Check sheet for the modelled part. Datum: model origin and axes. Units: mm. Face numbers are marked on the shaded views. A direction names the side the tool comes from. Coordinates: 2 decimals unless noted, no trailing zeros. Write each loop counter-clockwise with the first axis right and the second up, starting at its lowest first coordinate (ties: lowest second). Pieces come first, ordered by that corner, then holes. Notation, with made-up numbers: M 15.5,50.25 L 37.5,50.25 A25 ccw 37.5,88.25 Z; hole C 66,49 d4. An arc over 180 degrees is marked long. Answer as CSV lines item,"result". Start each with the question number.
1) Section check C-C (z = 3). Record the cut outline in (x, y), and give its area (3 significant figures).
2) Access from +Z, -Z, +X, -X, +Y, -Y to the whole of each face (thin tool, end or side, straight path). Record for the marked faces 1, 2 and 3.
3) Draft check along X on the marked faces 4, 5 and 6. Enter one of: +X half, -X half, draft (parallel to the pull), parting line (faces both ways), or undercut.
4) Go/stop test with flat-tipped pins: pin 1 Ø1 at (x, z) = (0.5, 3) entering from +Y; pin 2 Ø2 at (x, y) = (-2.5, 3) entering from +Z; pin 3 Ø1.2 at (x, y) = (0, 0) entering from +Z. Record where each tip stops, or that it passes through.
5) Section check A-A (y = 0). Record the cut outline in (x, z).
6) Material ranges on L1, parallel to Y at x = 0, z = 1.75; L2, parallel to Y at x = 0, z = 0.5, recorded low to high. Write a range as [from, to].
7) Section check D-D (y = -1.25). Record the cut outline in (x, z), and give its area (3 significant figures).
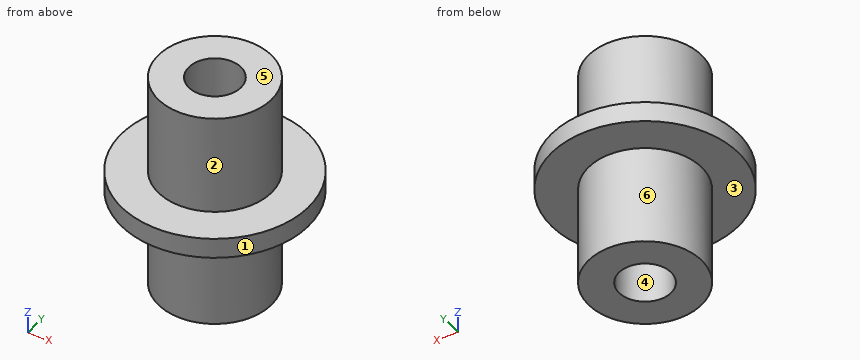
from build123d import *

# Parameters (mm, degrees)
F0_R     = 3.7338
F1_DEPTH = 0.8128
F2_R     = 2.2606
F3_DEPTH = 3.9878
F4_R     = 2.2606
F5_DEPTH = 3.9878
F6_R     = 1.0414
F7_DEPTH = 25.4


with BuildPart() as f1:
    # F0 (on Top) → F1 (new body)
    with BuildSketch(Plane.XY):
        Circle(F0_R)
    extrude(amount=F1_DEPTH)

    # F2 (on face) → F3 (join)
    with BuildSketch(Plane.XY.offset(0.8128)):
        Circle(F2_R)
    extrude(amount=F3_DEPTH)

    # F4 (on face) → F5 (join)
    with BuildSketch(Plane(origin=(0, 0, 0), x_dir=(1, 0, 0), z_dir=(0, 0, -1))):
        Circle(F4_R)
    extrude(amount=F5_DEPTH)

    # F6 (on face) → F7 (cut)
    with BuildSketch(Plane(origin=(0, 0, -3.9878), x_dir=(1, 0, 0), z_dir=(0, 0, -1))):
        Circle(F6_R)
    extrude(amount=-F7_DEPTH, mode=Mode.SUBTRACT)


solid = f1.part
Results found:
1,outline,"C 0,0 d4.52; hole C 0,0 d2.08"
1,area,"12.6 mm2"
2,face 1,"+Z, -Z"
2,face 2,"+Z"
2,face 3,"-Z"
3,face 4,"undercut"
3,face 5,"draft"
3,face 6,"parting line"
4,pin 1,"stops at y = 2.26"
4,pin 2,"stops at z = 0.81"
4,pin 3,"passes through"
5,outline,"M -3.73,0 L -2.26,0 L -2.26,-3.99 L -1.04,-3.99 L -1.04,4.8 L -2.26,4.8 L -2.26,0.81 L -3.73,0.81 Z; M 1.04,-3.99 L 2.26,-3.99 L 2.26,0 L 3.73,0 L 3.73,0.81 L 2.26,0.81 L 2.26,4.8 L 1.04,4.8 Z"
6,L1,"y = [-2.26, -1.04], [1.04, 2.26]"
6,L2,"y = [-3.73, -1.04], [1.04, 3.73]"
7,outline,"M -3.52,0 L -1.88,0 L -1.88,-3.99 L 1.88,-3.99 L 1.88,0 L 3.52,0 L 3.52,0.81 L 1.88,0.81 L 1.88,4.8 L -1.88,4.8 L -1.88,0.81 L -3.52,0.81 Z"
7,area,"35.8 mm2"
